Build history of the part. All positions in model axes, mm. Face numbers are marked on the shaded views. A direction names the side the tool comes from. Coordinates: 2 decimals unless noted, no trailing zeros. Loops run counter-clockwise (first coordinate to the right, second up) from the corner with the lowest first, then second, coordinate; pieces in that order, holes last.
Item 1: Cut at A-A (y = 30). List the corners of the cut face in (x, z), and give its area (3 significant figures).
Item 2: 3-axis set-ups, long thin cutter, end or side, ignore diameter. For the marked faces 4, 5 and 6: which of +Z, -Z, +X, -X, +Y, -Y reach the whole face in a straight line?
Item 3: Drill centre lines: line 1 along X through (y, z) = (16, 94); line 2 along Z through (x, y) = (46, 9.5); line 3 along X through (y, z) = (4.5, 100). Where is each one in solid material? Low to high.
Item 4: Cut at B-B (z = 13). List the corners of the cut face in (x, y), and give its area (3 significant figures).
Item 5: Flat gauge pins, fed straight in: pin 1 (8 mm diameter, centred on x = 59, y = 5, fed in from -Z); pin 2 (8 mm diameter, centred on y = 15.5, z = 77, fed in from +X); pin 3 (12 mm diameter, centred on x = 26.5, z = 51.5, fed in from -Y); pin 4 (22 mm diameter, centred on y = 9, z = 7, fed in from +X). Where does each tip first touch, or does it go through?
Item 6: Mould opens along Z. For the marked faces 1, 2 and 3 say: released by +Z, released by -Z, zero draft, split by the parting line, or undercut.
Item 7: Cut at C-C (x = 24.5). List the corners of the cut face in (y, z).
Item 8: Cut at D-D (x = 13.5). List the corners of the cut face in (y, z), and give its area (3 significant figures).
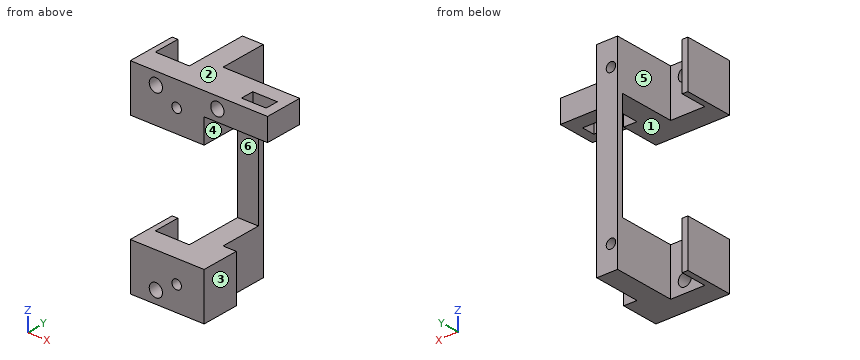
from build123d import *

# Parameters (mm, degrees)
SALIENTE_EXTRUIR1_DEPTH = 107
CROQUIS3_W              = 57
CROQUIS3_H              = 42
CORTAR_EXTRUIR1_DEPTH   = 39
CORTAR_EXTRUIR2_REACH   = 47
CROQUIS2_R              = 2.5
CORTAR_EXTRUIR3_REACH   = 14
CROQUIS4_R              = 3.5
CROQUIS5_W              = 12
CROQUIS5_H              = 20
SALIENTE_EXTRUIR2_DEPTH = 33.5
CORTAR_EXTRUIR4_REACH   = 22
CROQUIS7_R              = 3.5
CORTAR_EXTRUIR5_REACH   = 109
CROQUIS8_W              = 13
CROQUIS8_H              = 7


with BuildPart() as part:
    # Croquis1 → Saliente-Extruir1 (new body)
    with BuildSketch(Plane.XY):
        Polygon((0, 0), (39, 0), (39, 20), (32, 20), (32, 45), (21, 45), (21, 12), (3, 12), (3, 26), (0, 26), align=None)
    extrude(amount=SALIENTE_EXTRUIR1_DEPTH)

    # Croquis3 → Cortar-Extruir1 (cut)
    with BuildSketch(Plane.ZY):
        with Locations((53.5, 21)):
            Rectangle(CROQUIS3_W, CROQUIS3_H)
    extrude(amount=-CORTAR_EXTRUIR1_DEPTH, mode=Mode.SUBTRACT)

    # Croquis2 → Cortar-Extruir2 (cut, up to next)
    with BuildSketch(Plane(origin=(0, 45, 0), x_dir=(1, 0, 0), z_dir=(0, 1, 0)), mode=Mode.PRIVATE) as cortar_extruir2_sk1:
        with Locations((24.5, -94)):
            Circle(CROQUIS2_R)
    cortar_extruir2_tool1 = extrude(cortar_extruir2_sk1.sketch, amount=-CORTAR_EXTRUIR2_REACH, mode=Mode.PRIVATE) & part.part
    add(cortar_extruir2_tool1.solids().sort_by_distance((24.5, 45, 94))[0], mode=Mode.SUBTRACT)
    # Croquis2 → Cortar-Extruir2 (cut, up to next)
    with BuildSketch(Plane(origin=(0, 45, 0), x_dir=(1, 0, 0), z_dir=(0, 1, 0)), mode=Mode.PRIVATE) as cortar_extruir2_sk2:
        with Locations((24.5, -13)):
            Circle(CROQUIS2_R)
    cortar_extruir2_tool2 = extrude(cortar_extruir2_sk2.sketch, amount=-CORTAR_EXTRUIR2_REACH, mode=Mode.PRIVATE) & part.part
    add(cortar_extruir2_tool2.solids().sort_by_distance((24.5, 45, 13))[0], mode=Mode.SUBTRACT)

    # Croquis4 → Cortar-Extruir3 (cut, up to next)
    with BuildSketch(Plane(origin=(0, 12, 0), x_dir=(1, 0, 0), z_dir=(0, 1, 0)), mode=Mode.PRIVATE) as cortar_extruir3_sk1:
        with Locations((13.5, -100.5)):
            Circle(CROQUIS4_R)
    cortar_extruir3_tool1 = extrude(cortar_extruir3_sk1.sketch, amount=-CORTAR_EXTRUIR3_REACH, mode=Mode.PRIVATE) & part.part
    add(cortar_extruir3_tool1.solids().sort_by_distance((13.5, 12, 100.5))[0], mode=Mode.SUBTRACT)
    # Croquis4 → Cortar-Extruir3 (cut, up to next)
    with BuildSketch(Plane(origin=(0, 12, 0), x_dir=(1, 0, 0), z_dir=(0, 1, 0)), mode=Mode.PRIVATE) as cortar_extruir3_sk2:
        with Locations((13.5, -6.5)):
            Circle(CROQUIS4_R)
    cortar_extruir3_tool2 = extrude(cortar_extruir3_sk2.sketch, amount=-CORTAR_EXTRUIR3_REACH, mode=Mode.PRIVATE) & part.part
    add(cortar_extruir3_tool2.solids().sort_by_distance((13.5, 12, 6.5))[0], mode=Mode.SUBTRACT)

    # Croquis5 → Saliente-Extruir2 (add)
    with BuildSketch(Plane(origin=(39, 0, 0), x_dir=(0, 0, -1), z_dir=(1, 0, 0))):
        with Locations((-101, 10)):
            Rectangle(CROQUIS5_W, CROQUIS5_H)
    extrude(amount=SALIENTE_EXTRUIR2_DEPTH)

    # Croquis7 → Cortar-Extruir4 (cut, up to next)
    with BuildSketch(Plane(origin=(0, 20, 0), x_dir=(1, 0, 0), z_dir=(0, 1, 0)), mode=Mode.PRIVATE) as cortar_extruir4_sk1:
        with Locations((46, -101.053923336)):
            Circle(CROQUIS7_R)
    cortar_extruir4_tool1 = extrude(cortar_extruir4_sk1.sketch, amount=-CORTAR_EXTRUIR4_REACH, mode=Mode.PRIVATE) & part.part
    add(cortar_extruir4_tool1.solids().sort_by_distance((46, 20, 101.053923))[0], mode=Mode.SUBTRACT)

    # Croquis8 → Cortar-Extruir5 (cut, up to next)
    with BuildSketch(Plane.XY.offset(107), mode=Mode.PRIVATE) as cortar_extruir5_sk1:
        with Locations((61, 8.5)):
            Rectangle(CROQUIS8_W, CROQUIS8_H)
    cortar_extruir5_tool1 = extrude(cortar_extruir5_sk1.sketch, amount=-CORTAR_EXTRUIR5_REACH, mode=Mode.PRIVATE) & part.part
    add(cortar_extruir5_tool1.solids().sort_by_distance((61, 8.5, 107))[0], mode=Mode.SUBTRACT)


solid = part.part
Filled sheet:
1. outline: (21, 0) - (32, 0) - (32, 25) - (21, 25) - close; (21, 82) - (32, 82) - (32, 107) - (21, 107) - close; hole circle Ø5 at (24.5, 13); hole circle Ø5 at (24.5, 94)
1. area: 511 mm2
2. face 4: -Z, +X, +Y, -Y
2. face 5: +Z, -Z, +Y
2. face 6: +X, -X, -Y
3. line 1: x = 0 to 3, 21 to 22, 27 to 39
3. line 2: z = 95 to 97.55, 104.55 to 107
3. line 3: x = 0 to 10.04, 16.96 to 42.66, 49.34 to 72.5
4. outline: (0, 0) - (22, 0) - (22, 45) - (21, 45) - (21, 12) - (3, 12) - (3, 26) - (0, 26) - close; (27, 0) - (39, 0) - (39, 20) - (32, 20) - (32, 45) - (27, 45) - close
4. area: 704 mm2
5. pin 1: stops at z = 95
5. pin 2: passes through
5. pin 3: stops at y = 42
5. pin 4: stops at x = 39
6. face 1: undercut
6. face 2: released by +Z
6. face 3: zero draft
7. outline: (0, 0) - (45, 0) - (45, 10.5) - (0, 10.5) - close; (0, 15.5) - (45, 15.5) - (45, 91.5) - (0, 91.5) - (0, 82) - (42, 82) - (42, 25) - (0, 25) - close; (0, 96.5) - (45, 96.5) - (45, 107) - (0, 107) - close
8. outline: (0, 0) - (12, 0) - (12, 3) - (0, 3) - close; (0, 10) - (12, 10) - (12, 25) - (0, 25) - close; (0, 82) - (12, 82) - (12, 97) - (0, 97) - close; (0, 104) - (12, 104) - (12, 107) - (0, 107) - close
8. area: 432 mm2
